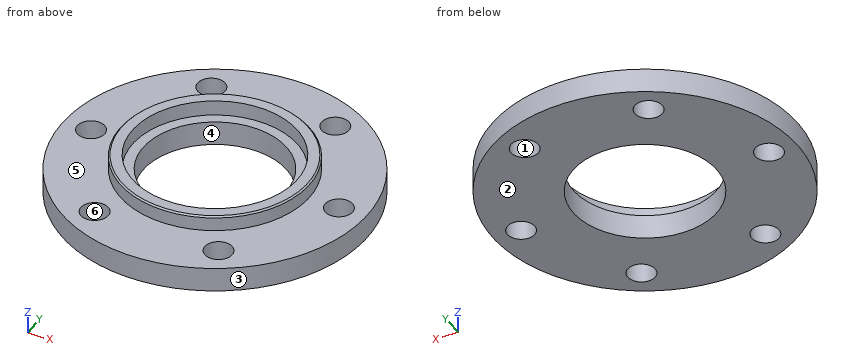
from build123d import *

# Parameters (mm, degrees)
SKETCH_1_R          = 50
EXTRUDE_1_DEPTH     = 8
SKETCH_2_R          = 31
EXTRUDE_2_DEPTH     = 5
SKETCH_3_R          = 27
CUT_EXTRUDE_2_DEPTH = 5
SKETCH_4_R          = 23.5
CUT_EXTRUDE_3_DEPTH = 72.161787499
SKETCH_5_R          = 4.5
CUT_EXTRUDE_4_DEPTH = 72.161787499
CHAMFER_1_SIZE      = 0.5


with BuildPart() as part:
    # 草图1 → 凸台-拉伸1 (new body)
    with BuildSketch(Plane.XY):
        Circle(SKETCH_1_R)
    extrude(amount=EXTRUDE_1_DEPTH)

    # 草图2 → 凸台-拉伸2 (add)
    with BuildSketch(Plane.XY.offset(8)):
        Circle(SKETCH_2_R)
    extrude(amount=EXTRUDE_2_DEPTH)

    # 草图3 → 切除-拉伸2 (cut)
    with BuildSketch(Plane.XY.offset(13)):
        Circle(SKETCH_3_R)
    extrude(amount=-CUT_EXTRUDE_2_DEPTH, mode=Mode.SUBTRACT)

    # 草图4 → 切除-拉伸3 (cut, through all)
    with BuildSketch(Plane.XY.offset(8)):
        Circle(SKETCH_4_R)
    extrude(amount=-CUT_EXTRUDE_3_DEPTH, mode=Mode.SUBTRACT)

    # 草图5 → 切除-拉伸4 (cut, through all)
    with BuildSketch(Plane.XY.offset(8)):
        with Locations((40.994281337, 0.684761001)):
            Circle(SKETCH_5_R)
        with Locations((21.090161091, -35.159708548)):
            Circle(SKETCH_5_R)
        with Locations((-19.904120246, -35.844469549)):
            Circle(SKETCH_5_R)
        with Locations((-40.994281337, -0.684761001)):
            Circle(SKETCH_5_R)
        with Locations((-21.090161091, 35.159708548)):
            Circle(SKETCH_5_R)
        with Locations((19.904120246, 35.844469549)):
            Circle(SKETCH_5_R)
    extrude(amount=-CUT_EXTRUDE_4_DEPTH, mode=Mode.SUBTRACT)

    # 倒角1
    chamfer_1_edges = [part.edges().sort_by_distance(p)[0] for p in [
        (-31, 0, 13),
    ]]
    chamfer(chamfer_1_edges, length=CHAMFER_1_SIZE)


solid = part.part
Design review of the part built by this model. Coordinates are the model's own, in mm. Face numbers are marked on the shaded views. A direction names the side the tool comes from. Round coordinates to 2 decimals unless told otherwise and drop trailing zeros. Write each loop counter-clockwise with the first axis right and the second up, starting at its lowest first coordinate (ties: lowest second). Pieces come first, ordered by that corner, then holes.
Item 1: For the marked faces 5 and 6, list the 3-axis set-ups (+Z, -Z, +X, -X, +Y, -Y) from which the entire face can be reached by the end or side of a thin tool; tool diameter is ignored.
Item 2: Consider section A-A on x = 0. Give the boundary of the cut face in (y, z), and give its area (3 significant figures).
Item 3: Draft analysis for pull direction Y (two halves, no side actions). For the marked faces 1, 2, 3 and 4, state which applies: released by +Y, released by -Y, zero draft, split by the parting line, or undercut.
Item 4: Consider section D-D on x = -39. Give the boundary of the cut face in (y, z).
Item 5: Consider section C-C on y = 38.5. Give the boundary of the cut face in (x, z), and give its area (3 significant figures).
Item 6: Wall thickness on L1, parallel to Y at x = 0, z = 2.5; L2, parallel to X at y = 32.5, z = 2; L3, parallel to Y at x = -8.5, z = 12: over which ranges is each line inside the solid? List them lowest first.
Item 7: Consider section B-B on z = 5.5. Give the boundary of the cut face in (x, y).
Item 8: For pin 1 Ø3 at (x, z) = (36, 2) entering from +Y; pin 2 Ø14.5 at (x, y) = (-21.09, 35.16) entering from -Z; pin 3 Ø5.5 at (x, y) = (21.09, -35.16) entering from +Z (1 decimal); pin 4 Ø2 at (x, z) = (16.5, 11.5) entering from +Y, all flat-tipped, find the tip position at first contact; note any pin that passes through.
Check values:
1. face 5: +Z
1. face 6: +Z, -Z
2. outline: (-50, 0) - (-23.5, 0) - (-23.5, 8) - (-27, 8) - (-27, 13) - (-30.5, 13) - (-31, 12.5) - (-31, 8) - (-50, 8) - close; (23.5, 0) - (50, 0) - (50, 8) - (31, 8) - (31, 12.5) - (30.5, 13) - (27, 13) - (27, 8) - (23.5, 8) - close
2. area: 464 mm2
3. face 1: undercut
3. face 2: zero draft
3. face 3: split by the parting line
3. face 4: undercut
4. outline: (-31.29, 0) - (-4.72, 0) - (-4.72, 8) - (-31.29, 8) - close; (3.35, 0) - (31.29, 0) - (31.29, 8) - (3.35, 8) - close
5. outline: (-31.9, 0) - (-24.11, 0) - (-24.11, 8) - (-31.9, 8) - close; (-18.07, 0) - (16.27, 0) - (16.27, 8) - (-18.07, 8) - close; (23.54, 0) - (31.9, 0) - (31.9, 8) - (23.54, 8) - close
5. area: 404 mm2
6. L1: y = -50 to -23.5, 23.5 to 50
6. L2: x = -38 to -24.72, -17.46 to 16.89, 22.91 to 38
6. L3: y = -29.81 to -25.63, 25.63 to 29.81
7. outline: circle Ø100 at (0, 0); hole circle Ø9 at (-40.99, -0.68); hole circle Ø9 at (-21.09, 35.16); hole circle Ø9 at (-19.9, -35.84); hole circle Ø47 at (0, 0); hole circle Ø9 at (19.9, 35.84); hole circle Ø9 at (21.09, -35.16); hole circle Ø9 at (40.99, 0.68)
8. pin 1: stops at y = 36.19
8. pin 2: stops at z = 0
8. pin 3: passes through
8. pin 4: stops at y = 26.85
